from build123d import *

# Parameters (mm, degrees)
V10_MIC_14X12P8_PCB_START               = -9
SKETCH_4_W                              = 14
SKETCH_4_H                              = 12.8
V10_MIC_14X12P8_PCB_DEPTH               = 1.6
V10_MIC_SOUND_PACKAGE_FACING_LID_START  = -7.4
SKETCH_5_W                              = 3
SKETCH_5_H                              = 4
V10_MIC_SOUND_PACKAGE_FACING_LID_DEPTH  = 1.2
SKETCH_6_R                              = 1.3
V10_MIC_REFERENCE_HOLES_PITCH8P89_DEPTH = 1.6


with BuildPart() as part:
    # 草图4 → V10_MIC_14x12p8_pcb (new body)
    with BuildSketch(Plane.XY.offset(V10_MIC_14X12P8_PCB_START)):
        with Locations((65, 33)):
            Rectangle(SKETCH_4_W, SKETCH_4_H)
    extrude(amount=V10_MIC_14X12P8_PCB_DEPTH)

    # 草图5 → V10_MIC_sound_package_facing_lid (add)
    with BuildSketch(Plane.XY.offset(V10_MIC_SOUND_PACKAGE_FACING_LID_START)):
        with Locations((65, 33)):
            Rectangle(SKETCH_5_W, SKETCH_5_H)
    extrude(amount=V10_MIC_SOUND_PACKAGE_FACING_LID_DEPTH)

    # 草图6 → V10_MIC_reference_holes_pitch8p89 (cut)
    with BuildSketch(Plane.XY.offset(-7.4)):
        with Locations((60.555, 36.81)):
            Circle(SKETCH_6_R)
        with Locations((69.445, 36.81)):
            Circle(SKETCH_6_R)
    extrude(amount=-V10_MIC_REFERENCE_HOLES_PITCH8P89_DEPTH, mode=Mode.SUBTRACT)


solid = part.part
Build history of the part. All positions in model axes, mm. A direction names the side the tool comes from. Give positions to 0.01 mm unless a question says otherwise; leave off trailing zeros. Write each loop counter-clockwise with the first axis right and the second up, starting at its lowest first coordinate (ties: lowest second). Pieces come first, ordered by that corner, then holes. Notation, with made-up numbers: (-28.5, 52.5) - (-11.5, 52.5) arc R21 ccw to (-11.5, 87.5) - close; hole circle Ø9 at (-36.75, 50.5). An arc over 180 degrees is marked (long way). Use one line per item in the form item = value. Start each with the question number.
1. Drop flat-ended pins along their axis: pin 1 Ø0.6 at (x, z) = (65, -7) entering from -Y; pin 2 Ø0.6 at (y, z) = (32, -7) entering from +X; pin 3 Ø2.5 at (x, y) = (60.555, 36.81) entering from +Z; pin 4 Ø0.6 at (x, z) = (64.5, -6.5) entering from +Y. Give the stop position or say it passes through.
2. Two-plate mould, pull along Y, no slides. Class faces 5 (the face through (65, 35, -7)), 6 (the face through (68.146, 36.867, -8.189)), 7 (the face through (63, 33, -7.4)): released by +Y, released by -Y, zero draft, split by the parting line, or undercut.
3. Band-saw the part on A-A on y = 34. Write the cut outline in (x, z).
4. Probe line 1 (X direction, y = 36.5, z = -8); line 2 (X direction, y = 31.5, z = -6.7); line 3 (Z direction, x = 67.5, y = 34.25). List the from-to ranges inside material, lowest first. Write a range as [from, to].
5. Band-saw the part on D-D on z = -6.9. Write the cut outline in (x, y), plus the area to 3 significant figures.
6. Band-saw the part on C-C on x = 69.5. Write the cut outline in (y, z), plus the area to 3 significant figures.
7. 3-axis set-ups, long thin cutter, end or side, ignore diameter. For faces 1 (the face through (65, 31, -7)), 2 (the face through (72, 33, -8)), 3 (the face through (63.5, 33, -7)), 4 (the face through (66.5, 33, -7)): which of +Z, -Z, +X, -X, +Y, -Y reach the whole face in a straight line?
8. Band-saw the part on B-B on y = 36.81. Write the cut outline in (x, z) (3 decimals), plus the area to 3 significant figures.
Conclusion:
q1.pin_1 = 31
q1.pin_2 = 66.5
q1.pin_3 = through
q1.pin_4 = 35
q2.face_5 = released by +Y
q2.face_6 = undercut
q2.face_7 = zero draft
q3.outline = (58, -9) - (72, -9) - (72, -7.4) - (66.5, -7.4) - (66.5, -6.2) - (63.5, -6.2) - (63.5, -7.4) - (58, -7.4) - close
q4.line_1 = [58, 59.29], [61.82, 68.18], [70.71, 72]
q4.line_2 = [63.5, 66.5]
q4.line_3 = [-9, -7.4]
q5.outline = (63.5, 31) - (66.5, 31) - (66.5, 35) - (63.5, 35) - close
q5.area = 12.0 mm²
q6.outline = (26.6, -9) - (35.51, -9) - (35.51, -7.4) - (26.6, -7.4) - close; (38.11, -9) - (39.4, -9) - (39.4, -7.4) - (38.11, -7.4) - close
q6.area = 16.3 mm²
q7.face_1 = +Z, +X, -X, -Y
q7.face_2 = +Z, -Z, +X, +Y, -Y
q7.face_3 = +Z, -X, +Y, -Y
q7.face_4 = +Z, +X, +Y, -Y
q8.outline = (58, -9) - (59.255, -9) - (59.255, -7.4) - (58, -7.4) - close; (61.855, -9) - (68.145, -9) - (68.145, -7.4) - (61.855, -7.4) - close; (70.745, -9) - (72, -9) - (72, -7.4) - (70.745, -7.4) - close
q8.area = 14.1 mm²
